from build123d import *

# Parameters (mm, degrees)
F0_R     = 1
F0_R_2   = 2.95
F1_DEPTH = 6


with BuildPart() as f1:
    # F0 (on Front) → F1 (new body, symmetric)
    with BuildSketch(Plane.XZ):
        with BuildLine():
            Line((19, -6.244998), (19, 6.244998))
            ThreePointArc((19, 6.244998), (-20, 0), (19, -6.244998))
        make_face()
        with Locations((0, -15)):
            Circle(F0_R, mode=Mode.SUBTRACT)
        Circle(F0_R_2, mode=Mode.SUBTRACT)
        with Locations((0, 15)):
            Circle(F0_R, mode=Mode.SUBTRACT)
    extrude(amount=F1_DEPTH, both=True)


solid = f1.part
Design review of the part built by this model. Coordinates are the model's own, in mm. Round coordinates to 2 decimals unless told otherwise and drop trailing zeros. Write each loop counter-clockwise with the first axis right and the second up, starting at its lowest first coordinate (ties: lowest second). Pieces come first, ordered by that corner, then holes. Notation, with made-up numbers: (15.5, -17) - (48.5, -17) arc R26 cw to (48.5, 8) - close; hole circle Ø6 at (-32, -9). An arc over 180 degrees is marked (long way). Return JSON: item names as keys, results as strings. Group by question number.
Item 1: For probe 1 along Z at (x, y) = (0, -2.75); probe 2 along Z at (x, y) = (-2.5, 4); probe 3 along X at (y, z) = (1.5, -11.5), list the stretches that pass through material, from the lowest coordinate up. Write a range as [from, to].
Item 2: We need section B-B on z = 15. Write out the cut boundary in (x, y).
Item 3: The part is to be moulded in two halves that separate along Z. For faces 1 (the face through (0, 0, 14)), 2 (the face through (-19.984, -0.084, 0.791)), 3 (the face through (4, 6, 0)), say which applies: pulls with the +Z half, pulls with the -Z half, needs draft (parallel to the pull), parting line crosses it, or undercut.
Item 4: Insertion check: P1, Ø4, axis at y = 0.5, z = -10.5, coming from the -X side; P2, Ø1, axis at y = 1.5, z = 7, coming from the +X side; P3, Ø2, axis at y = 0, z = -4, coming from the -X side; P4, Ø1.2, axis at x = 0, z = 15, coming from the +Y side. Each pin has a flat end and moves straight along its axis. Give the tip position at first contact, or say it passes through.
Item 5: We need section C-C on y = 3. Write out the cut boundary in (x, z) (3 decimals).
Item 6: We need section D-D on z = -12. Write out the cut boundary in (x, y), and give its area (3 significant figures).
Item 7: We need section A-A on x = 0. Write out the cut boundary in (y, z), and give its area (3 significant figures).
Model answer:
{
 "1": {"probe 1": "z = [-20, -16], [-14, -2.95], [2.95, 14], [16, 20]", "probe 2": "z = [-19.84, -1.57], [1.57, 19.84]", "probe 3": "x = [-16.36, 16.36]"},
 "2": {"outline": "(-13.23, -6) - (-1, -6) - (-1, 6) - (-13.23, 6) - close; (1, -6) - (13.23, -6) - (13.23, 6) - (1, 6) - close"},
 "3": {"face 1": "undercut", "face 2": "parting line crosses it", "face 3": "needs draft"},
 "4": {"P1": "stops at x = -18.1", "P2": "stops at x = 18.91", "P3": "stops at x = -19.77", "P4": "passes through"},
 "5": {"outline": "(19, -6.245) - (19, 6.245) arc R20 ccw (long way) to start; hole circle Ø5.9 at (0, 0); hole circle Ø2 at (0, -15); hole circle Ø2 at (0, 15)"},
 "6": {"outline": "(-16, -6) - (16, -6) - (16, 6) - (-16, 6) - close", "area": "384 mm²"},
 "7": {"outline": "(-6, -20) - (6, -20) - (6, -16) - (-6, -16) - close; (-6, -14) - (6, -14) - (6, -2.95) - (-6, -2.95) - close; (-6, 2.95) - (6, 2.95) - (6, 14) - (-6, 14) - close; (-6, 16) - (6, 16) - (6, 20) - (-6, 20) - close", "area": "361 mm²"}
}
